Geometry check sheet. Reference: the model listing, model coordinates, mm. Coordinates: 2 decimals unless noted, no trailing zeros. Loops run counter-clockwise (first coordinate to the right, second up) from the corner with the lowest first, then second, coordinate; pieces in that order, holes last.
from build123d import *

# Parameters (mm, degrees)
SKETCH1_W               = 76.2
SKETCH1_H               = 76.2
SKETCH1_R               = 31.75
BOSS_EXTRUDE1_DEPTH     = 1.5875
SKETCH2_R               = 3.572453457
CUT_EXTRUDE1_DEPTH      = 3.175
SKETCH5_W               = 38.678922036
SKETCH5_H               = 46.509488783
CUT_EXTRUDE3_DEPTH      = 2.5875
MIRROR2_COPY_1_SKETCH_R = 3.572453457
MIRROR2_COPY_1_DEPTH    = 3.175


with BuildPart() as part:
    # Sketch1 → Boss-Extrude1 (new body)
    with BuildSketch(Plane.XY):
        Rectangle(SKETCH1_W, SKETCH1_H)
        Circle(SKETCH1_R, mode=Mode.SUBTRACT)
    extrude(amount=BOSS_EXTRUDE1_DEPTH)

    # Sketch2 → Cut-Extrude1 (cut)
    with BuildSketch(Plane.XY.offset(1.5875)):
        with Locations((-31.75, 31.75)):
            Circle(SKETCH2_R)
    cut_extrude1 = extrude(amount=-CUT_EXTRUDE1_DEPTH, mode=Mode.SUBTRACT)

    # Sketch5 → Cut-Extrude3 (cut, through all)
    with BuildSketch(Plane.XY.offset(1.5875)):
        with Locations((0.289461018, 41.034744392)):
            Rectangle(SKETCH5_W, SKETCH5_H)
    extrude(amount=-CUT_EXTRUDE3_DEPTH, mode=Mode.SUBTRACT)

    # Mirror1: Cut-Extrude1 across plane
    add(cut_extrude1.mirror(Plane(origin=(0, 0, 0), x_dir=(0, 0, 1), z_dir=(1, 0, 0))), mode=Mode.SUBTRACT)

    # Mirror2: Cut-Extrude1 across plane
    add(cut_extrude1.mirror(Plane.ZX), mode=Mode.SUBTRACT)

    # Mirror2 copy 1 sketch → Mirror2 copy 1 (cut)
    with BuildSketch(Plane(origin=(0, 0, 1.5875), x_dir=(-1, 0, 0), z_dir=(0, 0, 1))):
        with Locations((-31.75, 31.75)):
            Circle(MIRROR2_COPY_1_SKETCH_R)
    extrude(amount=-MIRROR2_COPY_1_DEPTH, mode=Mode.SUBTRACT)


solid = part.part
1) Depth check by flat-ended pin: pin 1 (4.5 mm diameter, centred on x = -31.75, y = 31.75, fed in from -Z). Enter the tip coordinate at first touch or a pass-through.
Data:
pin 1: passes through
2) Section check A-A on y = 31.75. Record the cut outline in (x, z), and give its area (3 significant figures).
Data:
outline: (-38.1, 0) - (-35.32, 0) - (-35.32, 1.59) - (-38.1, 1.59) - close; (-28.18, 0) - (-19.05, 0) - (-19.05, 1.59) - (-28.18, 1.59) - close; (19.63, 0) - (28.18, 0) - (28.18, 1.59) - (19.63, 1.59) - close; (35.32, 0) - (38.1, 0) - (38.1, 1.59) - (35.32, 1.59) - close
area: 36.9 mm2
3) Section check D-D on x = 0. Record the cut outline in (y, z), and give its area (3 significant figures).
Data:
outline: (-38.1, 0) - (-31.75, 0) - (-31.75, 1.59) - (-38.1, 1.59) - close
area: 10.1 mm2
4) Material ranges on probe 1 along Y at (x, z) = (-28.5, 1.2); probe 2 along Y at (x, z) = (-33, 1.25); probe 3 along X at (y, z) = (0, 0.7), recorded low to high.
Data:
probe 1: y = -38.1 to -33.23, -30.27 to -13.99, 13.99 to 30.27, 33.23 to 38.1
probe 2: y = -38.1 to -35.1, -28.4 to 28.4, 35.1 to 38.1
probe 3: x = -38.1 to -31.75, 31.75 to 38.1
5) Mould release check, pull along X, two halves, no side actions. Record for faces 1 (the cylindrical face through (-28.34, -32.82, 0.8)), 2 (the flat face through (8, -31, 0)): +X half, -X half, draft (parallel to the pull), parting line (faces both ways), or undercut.
Data:
face 1: undercut
face 2: draft
6) Section check B-B on z = 1. Record the cut outline in (x, y), and give its area (3 significant figures).
Data:
outline: (-38.1, -38.1) - (38.1, -38.1) - (38.1, 38.1) - (19.63, 38.1) - (19.63, 24.96) arc R31.75 cw (long way) to (-19.05, 25.4) - (-19.05, 38.1) - (-38.1, 38.1) - close; hole circle Ø7.14 at (-31.75, -31.75); hole circle Ø7.14 at (-31.75, 31.75); hole circle Ø7.14 at (31.75, -31.75); hole circle Ø7.14 at (31.75, 31.75)
area: 2,150 mm2
7) Section check C-C on y = -26. Record the cut outline in (x, z).
Data:
outline: (-38.1, 0) - (-18.22, 0) - (-18.22, 1.59) - (-38.1, 1.59) - close; (18.22, 0) - (38.1, 0) - (38.1, 1.59) - (18.22, 1.59) - close
